The model under review builds one solid part; all positions refer to its coordinate system, in mm. Face numbers are marked on the shaded views. A direction names the side the tool comes from. Round coordinates to 2 decimals unless told otherwise and drop trailing zeros. Order: outer loops, then holes, each group sorted by start corner. A loop starts at its lowest first (then second) coordinate and runs counter-clockwise, first axis right, second up.
1) Consider section D-D (x = -76.2). Give the boundary of the cut face in (y, z), then the cut area to 3 significant figures.
2) To check wall thickness, follow L1, parallel to Y at x = 76.2, z = -32; L2, parallel to X at y = -101.5, z = -49; L3, parallel to Z at x = 71, y = -78.5. State the ranges of each line that lie inside material, in increasing order.
3) Consider section C-C (z = 3). Give the boundary of the cut face in (x, y).
4) Consider section B-B (z = -43). Give the boundary of the cut face in (x, y).
5) Mouldability with a two-part tool opening along Z and no side actions: class the marked faces 4, 5 and 6 as pulls with the +Z half, pulls with the -Z half, needs draft (parallel to the pull), parting line crosses it, or undercut.
6) Consider section A-A (y = -101.6). Give the boundary of the cut face in (x, z), then the cut area to 3 significant figures.
7) Machinability: for the marked faces 1, 2 and 3, which of the approach directions +Z, -Z, +X, -X, +Y, -Y give a long, thin tool a straight path to every point of the face, cutting with its end or side? Answer none if there is none.
8) Clearance check with flat-ended pins moving along their axes: P1, Ø11.5, axis at x = 76.2, y = -101.6, coming from the +Z side; P2, Ø7.5, axis at x = -76.2, y = -25.4, coming from the -Z side; P3, Ø1.5, axis at y = -114, z = 29.5, coming from the -X side. State where each tip first meets the part, or that it passes through.
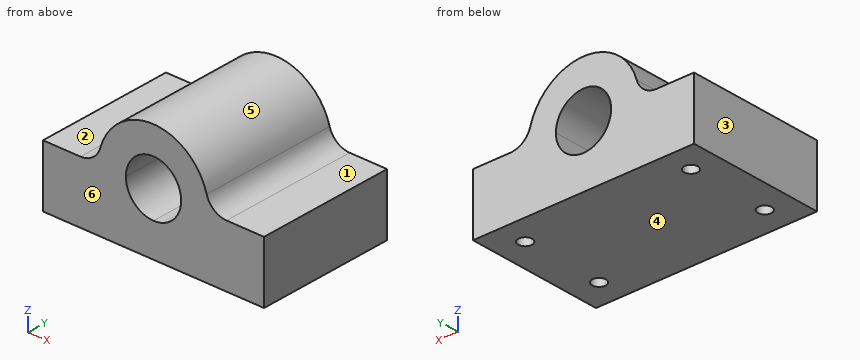
from build123d import *

# Parameters (mm, degrees)
F1_DEPTH = 127
F2_R     = 6.35
F3_DEPTH = 31.75


with BuildPart() as f1:
    # F0 (on Front) → F1 (new body)
    with BuildSketch(Plane.XZ):
        with BuildLine():
            Line((-101.6, -56.109019), (0, -56.109019))
            Line((0, -56.109019), (101.6, -56.109019))
            Line((101.6, -56.109019), (101.6, 0))
            Line((101.6, 0), (67.202083, 0))
            ThreePointArc((67.202083, 0), (55.714501, 3.853357), (48.874242, 13.854545))
            ThreePointArc((48.874242, 13.854545), (0, 50.8), (-48.874242, 13.854545))
            ThreePointArc((-48.874242, 13.854545), (-55.714501, 3.853357), (-67.202083, 0))
            Line((-67.202083, 0), (-101.6, 0))
            Line((-101.6, 0), (-101.6, -56.109019))
        make_face()
        with BuildLine():
            ThreePointArc((-25.4, 0), (0, 25.4), (25.4, 0))
            ThreePointArc((25.4, 0), (17.960512, -17.960512), (0, -25.4))
            ThreePointArc((0, -25.4), (-17.960512, -17.960512), (-25.4, 0))
        make_face(mode=Mode.SUBTRACT)
    extrude(amount=F1_DEPTH)

    # F2 (on face) → F3 (cut)
    with BuildSketch(Plane(origin=(0, 0, -56.109019), x_dir=(1, 0, 0), z_dir=(0, 0, -1))):
        with Locations((-76.2, 101.6)):
            Circle(F2_R)
        with Locations((-76.2, 25.4)):
            Circle(F2_R)
        with Locations((76.2, 101.6)):
            Circle(F2_R)
        with Locations((76.2, 25.4)):
            Circle(F2_R)
    extrude(amount=-F3_DEPTH, mode=Mode.SUBTRACT)


solid = f1.part
Answer below:
1. outline: (-127, -56.11) - (-107.95, -56.11) - (-107.95, -24.36) - (-95.25, -24.36) - (-95.25, -56.11) - (-31.75, -56.11) - (-31.75, -24.36) - (-19.05, -24.36) - (-19.05, -56.11) - (0, -56.11) - (0, 0) - (-127, 0) - close
1. area: 6,320 mm2
2. L1: y = -127 to -107.95, -95.25 to -31.75, -19.05 to 0
2. L2: x = -101.6 to -82.55, -69.85 to 69.85, 82.55 to 101.6
2. L3: z = -56.11 to 0
3. outline: (-56.94, -127) - (-25.22, -127) - (-25.22, 0) - (-56.94, 0) - close; (25.22, -127) - (56.94, -127) - (56.94, 0) - (25.22, 0) - close
4. outline: (-101.6, -127) - (101.6, -127) - (101.6, 0) - (-101.6, 0) - close; hole circle Ø12.7 at (-76.2, -101.6); hole circle Ø12.7 at (-76.2, -25.4); hole circle Ø12.7 at (76.2, -101.6); hole circle Ø12.7 at (76.2, -25.4)
5. face 4: pulls with the -Z half
5. face 5: pulls with the +Z half
5. face 6: needs draft
6. outline: (-101.6, -56.11) - (-82.55, -56.11) - (-82.55, -24.36) - (-69.85, -24.36) - (-69.85, -56.11) - (69.85, -56.11) - (69.85, -24.36) - (82.55, -24.36) - (82.55, -56.11) - (101.6, -56.11) - (101.6, 0) - (67.2, 0) arc R19.05 cw to (48.87, 13.85) arc R50.8 ccw to (-48.87, 13.85) arc R19.05 cw to (-67.2, 0) - (-101.6, 0) - close; hole circle Ø50.8 at (0, 0)
6. area: 12,700 mm2
7. face 1: +Z, +X, +Y, -Y
7. face 2: +Z, -X, +Y, -Y
7. face 3: +Z, -Z, -X, +Y, -Y
8. P1: stops at z = 0
8. P2: stops at z = -24.36
8. P3: stops at x = -41.88
